```python
from build123d import *

# Parameters (mm, degrees)
SKETCH1_R           = 2.1
BOSS_EXTRUDE1_DEPTH = 738


with BuildPart() as part:
    # Sketch1 → Boss-Extrude1 (new body)
    with BuildSketch(Plane.XY):
        with BuildLine():
            Line((4.58, -20), (9.5, -20))
            ThreePointArc((9.5, -20), (9.853553391, -19.853553391), (10, -19.5))
            Line((10, -19.5), (10, -14.58))
            Line((10, -14.58), (8.545, -13.125))
            Line((8.545, -13.125), (8.2, -13.125))
            Line((8.2, -13.125), (8.2, -15.5))
            Line((8.2, -15.5), (6.560660172, -15.5))
            Line((6.560660172, -15.5), (3.9, -12.839339828))
            Line((3.9, -12.839339828), (3.9, -10.21))
            Line((3.9, -10.21), (3.69, -10))
            Line((3.69, -10), (3.9, -9.79))
            Line((3.9, -9.79), (3.9, -7.160660172))
            Line((3.9, -7.160660172), (6.560660172, -4.5))
            Line((6.560660172, -4.5), (8.2, -4.5))
            Line((8.2, -4.5), (8.2, -6.875))
            Line((8.2, -6.875), (8.545, -6.875))
            Line((8.545, -6.875), (10, -5.42))
            Line((10, -5.42), (10, 5.42))
            Line((10, 5.42), (8.545, 6.875))
            Line((8.545, 6.875), (8.2, 6.875))
            Line((8.2, 6.875), (8.2, 4.5))
            Line((8.2, 4.5), (6.560660172, 4.5))
            Line((6.560660172, 4.5), (3.9, 7.160660172))
            Line((3.9, 7.160660172), (3.9, 9.79))
            Line((3.9, 9.79), (3.69, 10))
            Line((3.69, 10), (3.9, 10.21))
            Line((3.9, 10.21), (3.9, 12.839339828))
            Line((3.9, 12.839339828), (6.560660172, 15.5))
            Line((6.560660172, 15.5), (8.2, 15.5))
            Line((8.2, 15.5), (8.2, 13.125))
            Line((8.2, 13.125), (8.545, 13.125))
            Line((8.545, 13.125), (10, 14.58))
            Line((10, 14.58), (10, 19.5))
            ThreePointArc((10, 19.5), (9.853553391, 19.853553391), (9.5, 20))
            Line((9.5, 20), (4.58, 20))
            Line((4.58, 20), (3.125, 18.545))
            Line((3.125, 18.545), (3.125, 18.2))
            Line((3.125, 18.2), (5.5, 18.2))
            Line((5.5, 18.2), (5.5, 16.560660172))
            Line((5.5, 16.560660172), (2.839339828, 13.9))
            Line((2.839339828, 13.9), (0.21, 13.9))
            Line((0.21, 13.9), (0, 13.69))
            Line((0, 13.69), (-0.21, 13.9))
            Line((-0.21, 13.9), (-2.839339828, 13.9))
            Line((-2.839339828, 13.9), (-5.5, 16.560660172))
            Line((-5.5, 16.560660172), (-5.5, 18.2))
            Line((-5.5, 18.2), (-3.125, 18.2))
            Line((-3.125, 18.2), (-3.125, 18.545))
            Line((-3.125, 18.545), (-4.58, 20))
            Line((-4.58, 20), (-9.5, 20))
            ThreePointArc((-9.5, 20), (-9.853553391, 19.853553391), (-10, 19.5))
            Line((-10, 19.5), (-10, 14.58))
            Line((-10, 14.58), (-8.545, 13.125))
            Line((-8.545, 13.125), (-8.2, 13.125))
            Line((-8.2, 13.125), (-8.2, 15.5))
            Line((-8.2, 15.5), (-6.560660172, 15.5))
            Line((-6.560660172, 15.5), (-3.9, 12.839339828))
            Line((-3.9, 12.839339828), (-3.9, 10.21))
            Line((-3.9, 10.21), (-3.69, 10))
            Line((-3.69, 10), (-3.9, 9.79))
            Line((-3.9, 9.79), (-3.9, 7.160660172))
            Line((-3.9, 7.160660172), (-6.560660172, 4.5))
            Line((-6.560660172, 4.5), (-8.2, 4.5))
            Line((-8.2, 4.5), (-8.2, 6.875))
            Line((-8.2, 6.875), (-8.545, 6.875))
            Line((-8.545, 6.875), (-10, 5.42))
            Line((-10, 5.42), (-10, -5.42))
            Line((-10, -5.42), (-8.545, -6.875))
            Line((-8.545, -6.875), (-8.2, -6.875))
            Line((-8.2, -6.875), (-8.2, -4.5))
            Line((-8.2, -4.5), (-6.560660172, -4.5))
            Line((-6.560660172, -4.5), (-3.9, -7.160660172))
            Line((-3.9, -7.160660172), (-3.9, -9.79))
            Line((-3.9, -9.79), (-3.69, -10))
            Line((-3.69, -10), (-3.9, -10.21))
            Line((-3.9, -10.21), (-3.9, -12.839339828))
            Line((-3.9, -12.839339828), (-6.560660172, -15.5))
            Line((-6.560660172, -15.5), (-8.2, -15.5))
            Line((-8.2, -15.5), (-8.2, -13.125))
            Line((-8.2, -13.125), (-8.545, -13.125))
            Line((-8.545, -13.125), (-10, -14.58))
            Line((-10, -14.58), (-10, -19.5))
            ThreePointArc((-10, -19.5), (-9.853553391, -19.853553391), (-9.5, -20))
            Line((-9.5, -20), (-4.58, -20))
            Line((-4.58, -20), (-3.125, -18.545))
            Line((-3.125, -18.545), (-3.125, -18.2))
            Line((-3.125, -18.2), (-5.5, -18.2))
            Line((-5.5, -18.2), (-5.5, -16.560660172))
            Line((-5.5, -16.560660172), (-2.839339828, -13.9))
            Line((-2.839339828, -13.9), (-0.21, -13.9))
            Line((-0.21, -13.9), (0, -13.69))
            Line((0, -13.69), (0.21, -13.9))
            Line((0.21, -13.9), (2.839339828, -13.9))
            Line((2.839339828, -13.9), (5.5, -16.560660172))
            Line((5.5, -16.560660172), (5.5, -18.2))
            Line((5.5, -18.2), (3.125, -18.2))
            Line((3.125, -18.2), (3.125, -18.545))
            Line((3.125, -18.545), (4.58, -20))
        make_face()
        with Locations((0, -10)):
            Circle(SKETCH1_R, mode=Mode.SUBTRACT)
        Polygon((-6.239339828, -2.7), (-8.2, -2.7), (-8.2, 2.7), (-6.239339828, 2.7), (-2.839339828, 6.1), (2.839339828, 6.1), (6.239339828, 2.7), (8.2, 2.7), (8.2, -2.7), (6.239339828, -2.7), (2.839339828, -6.1), (-2.839339828, -6.1), align=None, mode=Mode.SUBTRACT)
        with Locations((0, 10)):
            Circle(SKETCH1_R, mode=Mode.SUBTRACT)
    extrude(amount=BOSS_EXTRUDE1_DEPTH)


solid = part.part
```
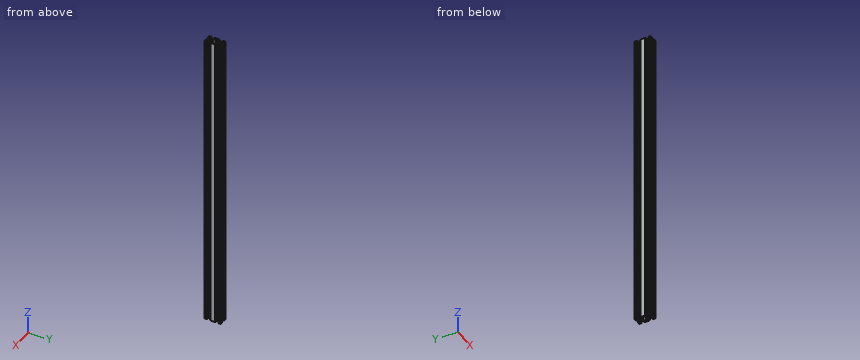
Source: CAD feature listing. Evaluate the final solid. Frame: model axes, mm. Round coordinates to 2 decimals unless told otherwise and drop trailing zeros. Answer as a JSON object with one key per item and string values. Group by question number.
(1) Section query A-A on z = 205. State how many separate pieces and enclosed holes the cut face has, then the cut area to 3 significant figures.
(2) First-contact query: pin 1 (1 mm diameter, centred on x = 5.5, y = -2.5, fed in from -Z); pin 2 (3 mm diameter, centred on y = 7, z = 634.5, fed in from +X); pin 3 (1.3 mm diameter, centred on y = -8, z = 484, fed in from +X). Flat tips, straight axial feed; report the tip coordinate or a pass-through.
(3) Ray query, line 1 (Y direction, x = 8, z = 686.5); line 2 (X direction, y = 5, z = 176); line 3 (Y direction, x = 8.5, z = 630.5) (3 decimals). Return the intervals inside material, ascending. Write a range as [from, to].
Computed values:
{
 "1": {"separate pieces": "1", "enclosed holes": "3", "area": "300 mm^2"},
 "2": {"pin 1": "through", "pin 2": "x = 9.92", "pin 3": "x = 3.9"},
 "3": {"line 1": "[-20, -15.5], [-4.5, -2.7], [2.7, 4.5], [15.5, 20]", "line 2": "[-10, -8.2], [-6.06, -3.94], [3.94, 6.06], [8.2, 10]", "line 3": "[-20, -13.125], [-6.875, 6.875], [13.125, 20]"}
}
